from build123d import *

# Parameters (mm, degrees)
CUT_EXTRUDE1_START = 10
CUT_EXTRUDE1_DEPTH = 10
CIRPATTERN1_COUNT  = 16


with BuildPart() as part:
    # Sketch1 → Revolve1 (revolve)
    with BuildSketch(Plane(origin=(0, 0, 0), x_dir=(-1, 0, 0), z_dir=(0, 1, 0))):
        Polygon((1.5, 12.5), (1.5, 0), (6.5, 0), (6.5, 1.25), (4.838958179, 1.25), (4.838958179, 11.25), (6.5, 11.25), (6.5, 12.5), align=None)
    revolve(axis=Axis((0, 0, 0), (0, 0, 1)))

    # Sketch2 → Cut-Extrude1 (cut)
    with BuildSketch(Plane.XY.offset(1.25).offset(CUT_EXTRUDE1_START)):
        with BuildLine():
            ThreePointArc((-0.749588485, 4.780547391), (-0.63859776, 4.754009655), (-0.578400192, 4.657058919))
            ThreePointArc((-0.578400192, 4.657058919), (-0.550810767, 4.537510728), (-0.508789197, 4.422240897))
            ThreePointArc((-0.508789197, 4.422240897), (0, 4.088958179), (0.508789197, 4.422240897))
            ThreePointArc((0.508789197, 4.422240897), (0.550810767, 4.537510728), (0.578400192, 4.657058919))
            ThreePointArc((0.578400192, 4.657058919), (0.63859776, 4.754009655), (0.749588485, 4.780547391))
            ThreePointArc((0.749588485, 4.780547391), (0, 4.838958179), (-0.749588485, 4.780547391))
        make_face()
    cut_extrude1 = extrude(amount=-CUT_EXTRUDE1_DEPTH, mode=Mode.SUBTRACT)

    # CirPattern1: Cut-Extrude1 ×16 about axis
    cirpattern1_axis = Axis((0, 0, 0), (0, 0, 1))
    for i in range(1, CIRPATTERN1_COUNT):
        add(cut_extrude1.rotate(cirpattern1_axis, i * 360 / CIRPATTERN1_COUNT), mode=Mode.SUBTRACT)


solid = part.part
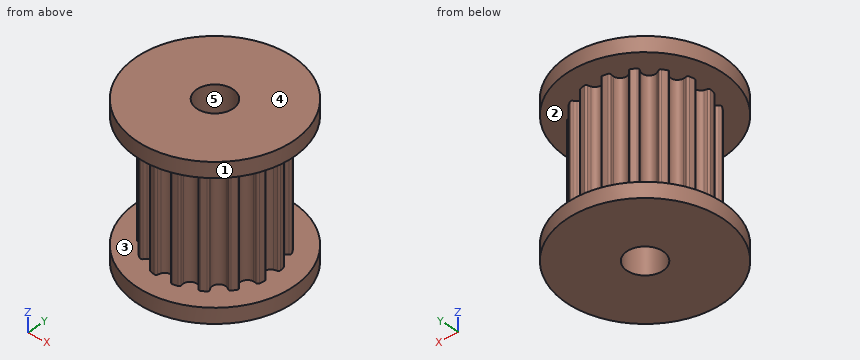
Model file for the job. Use its own axes, mm. Face numbers are marked on the shaded views. A direction names the side the tool comes from. Coordinates: 2 decimals unless noted, no trailing zeros. Order: outer loops, then holes, each group sorted by start corner. A loop starts at its lowest first (then second) coordinate and runs counter-clockwise, first axis right, second up. Notation, with made-up numbers: (-32.75, -25) -> (16.25, -25) arc R35 cw to (16.25, 12) -> close; hole circle Ø11 at (32, -23). An arc over 180 degrees is marked (long way). Return JSON: item names as keys, results as strings. Group by question number.
Item 1: Saw through at A-A on y = 0. Write the cut outline in (x, z), then the cut area to 3 significant figures.
Item 2: Tool access for the marked faces 1 and 2: list every direction of +Z, -Z, +X, -X, +Y, -Y with a clear straight run to the whole face (end or side of a thin tool).
Item 3: Flat gauge pins, fed straight in: P1, Ø1, axis at y = 3.5, z = 2, coming from the -X side; P2, Ø3, axis at y = 5, z = 5, coming from the +X side. Where does each tip first touch, or does it go through?
Item 4: Wall check: line 1 along Y through (x, z) = (0, 4); line 2 along Z through (x, y) = (-3.25, 5.5); line 3 along Y through (x, z) = (-3.5, 5.5). Give the ranges that are in metal, low to high. Write a range as [from, to].
Item 5: Pull direction Z, two halves, no side cores. Call the marked faces 3, 4 and 5: pulls with the +Z half, pulls with the -Z half, needs draft (parallel to the pull), parting line crosses it, or undercut.
Values found:
{
 "1": {"outline": "(-6.5, 0) -> (-1.5, 0) -> (-1.5, 12.5) -> (-6.5, 12.5) -> (-6.5, 11.25) -> (-4.09, 11.25) -> (-4.09, 1.25) -> (-6.5, 1.25) -> close; (1.5, 0) -> (6.5, 0) -> (6.5, 1.25) -> (4.09, 1.25) -> (4.09, 11.25) -> (6.5, 11.25) -> (6.5, 12.5) -> (1.5, 12.5) -> close", "area": "76.8 mm2"},
 "2": {"face 1": "+Z, -Z", "face 2": "none"},
 "3": {"P1": "stops at x = -2.91", "P2": "stops at x = 2.91"},
 "4": {"line 1": "y = [-4.09, -1.5], [1.5, 4.09]", "line 2": "z = [0, 1.25], [11.25, 12.5]", "line 3": "y = [-2.77, 2.77]"},
 "5": {"face 3": "undercut", "face 4": "pulls with the +Z half", "face 5": "needs draft"}
}
